from build123d import *

# Parameters (mm, degrees)
SKETCH1_R                = 140
SKETCH1_R_2              = 97
BOSS_EXTRUDE1_DEPTH      = 225
SKETCH3_R                = 23.5
BOSS_EXTRUDE3_DEPTH      = 32
CIRPATTERN1_COUNT        = 3
MIRROR1_COPY_1_SKETCH_R  = 23.5
MIRROR1_COPY_1_DEPTH     = 32
MIRROR1_COPY_2_SKETCH_R  = 23.5
MIRROR1_COPY_2_DEPTH     = 32
BOSS_EXTRUDE4_REACH      = 491.361
BOSS_EXTRUDE4_END_RADIUS = 140
SKETCH4_R                = 100
SKETCH5_R                = 50
CUT_EXTRUDE1_DEPTH       = 25
SKETCH6_R                = 25
CUT_EXTRUDE2_DEPTH       = 490.361006427
SKETCH7_R                = 12
CUT_EXTRUDE3_DEPTH       = 15


with BuildPart() as part:
    # Sketch1 → Boss-Extrude1 (new body)
    with BuildSketch(Plane(origin=(0, 0, 0), x_dir=(1, 0, 0), z_dir=(0, 1, 0))):
        with Locations(Location((0, 0, 0), (0, 0, 270))):
            Circle(SKETCH1_R)
        with Locations(Location((0, 0, 0), (0, 0, 270))):
            Circle(SKETCH1_R_2, mode=Mode.SUBTRACT)
    extrude(amount=BOSS_EXTRUDE1_DEPTH)

    # Sketch3 → Boss-Extrude3 (add)
    with BuildSketch(Plane(origin=(0, 225, 0), x_dir=(1, 0, 0), z_dir=(0, 1, 0))):
        with BuildLine():
            Line((-50, 175), (-50, 101.528699727))
            Line((-50, 101.528699727), (50, 101.528699727))
            Line((50, 101.528699727), (50, 175))
            ThreePointArc((50, 175), (0, 225), (-50, 175))
        make_face()
        with Locations(Location((0, 177.702584928, 0), (0, 0, 270))):
            Circle(SKETCH3_R, mode=Mode.SUBTRACT)
    boss_extrude3 = extrude(amount=-BOSS_EXTRUDE3_DEPTH)

    # CirPattern1: Boss-Extrude3 ×3 about axis
    cirpattern1_axis = Axis((0, 0, 0), (0, 1, 0))
    for i in range(1, CIRPATTERN1_COUNT):
        add(boss_extrude3.rotate(cirpattern1_axis, i * 360 / CIRPATTERN1_COUNT))

    # Mirror1: Boss-Extrude3 across plane
    add(boss_extrude3.mirror(Plane.ZX.offset(112.5)))

    # Mirror1 copy 1 sketch → Mirror1 copy 1 (add)
    with BuildSketch(Plane(origin=(0, 0, 0), x_dir=(-0.4999999999999998, 0, -0.8660254037844387), z_dir=(0, -1, 0))):
        with BuildLine():
            Line((-50, -175), (-50, -101.528699727))
            Line((-50, -101.528699727), (50, -101.528699727))
            Line((50, -101.528699727), (50, -175))
            ThreePointArc((50, -175), (0, -225), (-50, -175))
        make_face()
        with Locations((0, -177.702584928)):
            Circle(MIRROR1_COPY_1_SKETCH_R, mode=Mode.SUBTRACT)
    extrude(amount=-MIRROR1_COPY_1_DEPTH)

    # Mirror1 copy 2 sketch → Mirror1 copy 2 (add)
    with BuildSketch(Plane(origin=(0, 0, 0), x_dir=(-0.5000000000000004, 0, 0.8660254037844384), z_dir=(0, -1, 0))):
        with BuildLine():
            Line((-50, -175), (-50, -101.528699727))
            Line((-50, -101.528699727), (50, -101.528699727))
            Line((50, -101.528699727), (50, -175))
            ThreePointArc((50, -175), (0, -225), (-50, -175))
        make_face()
        with Locations((0, -177.702584928)):
            Circle(MIRROR1_COPY_2_SKETCH_R, mode=Mode.SUBTRACT)
    extrude(amount=-MIRROR1_COPY_2_DEPTH)

    # Boss-Extrude4: up to this cylinder (the profile starts outside it)
    boss_extrude4_end = Plane(origin=(0, 112.5, 0), z_dir=(0, -1, 0)) * Cylinder(BOSS_EXTRUDE4_END_RADIUS, 1263.722, mode=Mode.PRIVATE)
    # Sketch4 → Boss-Extrude4 (add, up to the surface)
    with BuildSketch(Plane.XY.offset(160), mode=Mode.PRIVATE) as boss_extrude4_sk1:
        with Locations((0, 112.5)):
            Circle(SKETCH4_R)
    boss_extrude4_tool1 = extrude(boss_extrude4_sk1.sketch, amount=-BOSS_EXTRUDE4_REACH, mode=Mode.PRIVATE) - boss_extrude4_end
    add(boss_extrude4_tool1.solids().sort_by_distance((0, 112.5, 160))[0])

    # Sketch5 → Cut-Extrude1 (cut)
    with BuildSketch(Plane.XY.offset(160)):
        with Locations((0, 112.5)):
            Circle(SKETCH5_R)
    extrude(amount=-CUT_EXTRUDE1_DEPTH, mode=Mode.SUBTRACT)

    # Sketch6 → Cut-Extrude2 (cut, through all)
    with BuildSketch(Plane.XY.offset(160)):
        with Locations((0, 112.5)):
            Circle(SKETCH6_R)
    extrude(amount=-CUT_EXTRUDE2_DEPTH, mode=Mode.SUBTRACT)

    # Sketch7 → Cut-Extrude3 (cut)
    with BuildSketch(Plane.XY.offset(160)):
        with Locations((0, 187.5)):
            Circle(SKETCH7_R)
        with Locations((64.951905284, 75)):
            Circle(SKETCH7_R)
        with Locations((-64.951905284, 75)):
            Circle(SKETCH7_R)
    extrude(amount=-CUT_EXTRUDE3_DEPTH, mode=Mode.SUBTRACT)


solid = part.part
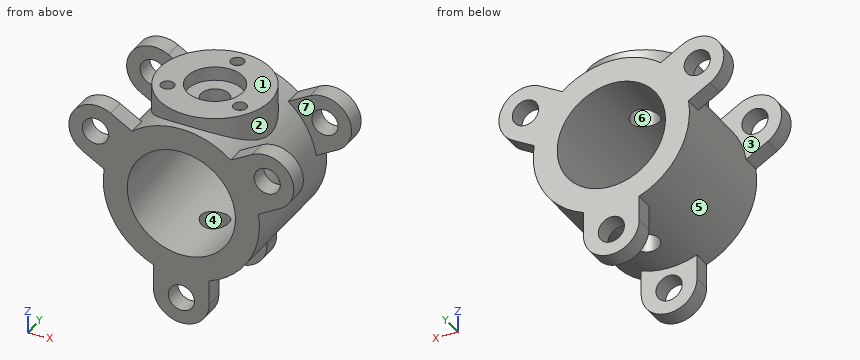
For this review, take the finished solid that the model builds, in its own axes (mm). Face numbers are marked on the shaded views. A direction names the side the tool comes from. Coordinates: 2 decimals unless noted, no trailing zeros. Loops run counter-clockwise (first coordinate to the right, second up) from the corner with the lowest first, then second, coordinate; pieces in that order, holes last. Notation, with made-up numbers: (17, -14.75) - (76, -14.75) arc R21 cw to (76, 9.25) - close; hole circle Ø9 at (49.5, -29.5). An arc over 180 degrees is marked (long way). Use a Markdown table: item, result. Add a question column.
Item 1: Insertion check: pin 1 Ø2 at (x, y) = (-114.5, 65) entering from +Z; pin 2 Ø21.5 at (x, y) = (64.95, 75) entering from +Z; pin 3 Ø2 at (x, y) = (0, 137.5) entering from -Z. Each pin has a flat end and moves straight along its axis. Give the tip position at first contact, or say it passes through.
Item 2: We need section C-C (x = -149). Give the boundary of the cut face in (y, z).
Item 3: Mouldability with a two-part tool opening along X and no side actions: class the marked faces 6 and 7 as pulls with the +X half, pulls with the -X half, needs draft (parallel to the pull), parting line crosses it, or undercut.
Item 4: We need section A-A (y = 122.5). Give the boundary of the cut face in (x, z).
Item 5: For line 1 (Y direction, x = 0, z = 123); line 2 (Z direction, x = 30.5, y = 180); line 3 (X direction, y = 211, z = 32), list the stretches that pass through material, from the lowest coordinate up.
Item 6: We need section B-B (z = -8.5). Give the boundary of the cut face in (x, y), and give its area (3 significant figures).
Item 7: Tool access review of the marked faces 1, 2, 3, 4 and 5: name each direction out of +Z, -Z, +X, -X, +Y, -Y from which nothing blocks a thin tool from reaching the whole face with its end or side.
Item 8: We need section D-D (z = -109). Give the boundary of the cut face in (x, y), and give its area (3 significant figures).
Results list:
| question | item | result |
|---|---|---|
| 1 | pin 1 | stops at z = 81.96 |
| 1 | pin 2 | stops at z = 145 |
| 1 | pin 3 | stops at z = -140 |
| 2 | outline | (0, 28.29) - (32, 28.29) - (32, 65.87) - (0, 65.87) - close; (0, 111.84) - (32, 111.84) - (32, 137.43) - (0, 137.43) - close; (193, 28.29) - (225, 28.29) - (225, 65.87) - (193, 65.87) - close; (193, 111.84) - (225, 111.84) - (225, 137.43) - (193, 137.43) - close |
| 3 | face 6 | undercut |
| 3 | face 7 | needs draft |
| 4 | outline | (-99.5, 98.49) arc R140 ccw to (-22.91, -138.11) - (-22.91, -94.25) arc R97 cw to (-22.91, 94.25) - (-22.91, 135) - (-48.99, 135) - (-48.99, 160) - (-99.5, 160) - close; (22.91, -138.11) arc R140 ccw to (99.5, 98.49) - (99.5, 160) - (48.99, 160) - (48.99, 135) - (22.91, 135) - (22.91, 94.25) arc R97 cw to (22.91, -94.25) - close |
| 5 | line 1 | y = 0 to 87.5, 137.5 to 225 |
| 5 | line 2 | z = -136.64 to -92.08, 92.08 to 160 |
| 5 | line 3 | x = -155.43 to -91.57, 91.57 to 155.43 |
| 6 | outline | (-139.74, 0) - (-96.63, 0) - (-96.63, 225) - (-139.74, 225) - close; (96.63, 0) - (139.74, 0) - (139.74, 225) - (96.63, 225) - close |
| 6 | area | 19,400 mm^2 |
| 7 | face 1 | +Z, +X, -X, +Y, -Y |
| 7 | face 2 | +Z |
| 7 | face 3 | +Z, -X |
| 7 | face 4 | +Z, -Z |
| 7 | face 5 | none |
| 8 | outline | (-87.86, 0) - (87.86, 0) - (87.86, 225) - (-87.86, 225) - close; hole circle Ø50 at (0, 112.5) |
| 8 | area | 37,600 mm^2 |
